Design review of the part built by this model. Coordinates are the model's own, in mm. Give positions to 0.01 mm unless a question says otherwise; leave off trailing zeros. Write each loop counter-clockwise with the first axis right and the second up, starting at its lowest first coordinate (ties: lowest second). Pieces come first, ordered by that corner, then holes. Notation, with made-up numbers: (14.25, -3.5) -> (67.25, -3.5) arc R18 ccw to (67.25, 31.5) -> close; hole circle Ø2 at (5, 9). An arc over 180 degrees is marked (long way). Return JSON: item names as keys, results as strings. Group by question number.
Autodesk Inventor part; units mm, degrees
ref_plane "YZ Plane" through (0, 0, 0) normal (1, 0, 0) x (0, 1, 0)
ref_plane "XZ Plane" through (0, 0, 0) normal (0, 1, 0) x (-1, 0, 0)
ref_plane "XY Plane" through (0, 0, 0) normal (0, 0, 1) x (1, 0, 0)
sketch "Sketch1" plane through (0, 0, 0) normal (0, 0, 1) x (1, 0, 0)
  line L0 (12.7, -4.7625) -> (-12.7, -4.7625)
  line L1 (-12.7, -4.7625) -> (-12.7, 4.7625)
  line L2 (-12.7, 4.7625) -> (12.7, 4.7625)
  line L3 (12.7, 4.7625) -> (12.7, -4.7625)
  line L4 (12.7, -4.7625) -> (-12.7, 4.7625) construction
  line L5 (-12.7, -4.7625) -> (12.7, 4.7625) construction
  line L6 (-12.7, 0) -> (12.7, 0) construction
  circle A0 centre (-7.1437, 0) radius 2.4892
  line L7 (0, -4.7625) -> (0, 4.7625) construction
  circle A1 centre (7.1437, 0) radius 2.4892
  point P0 (0, 0)
  point P1 (0, 0)
  dimension "d0" = 25.4
  dimension "d1" = 9.525
  dimension "d2" = 4.9784
  dimension "d3" = 7.1437
extrude "Extrusion1" add sketch "Sketch1" along normal blind 6.35
properties part number "Arms" material "Aluminum 6061"
Q1. Take a section at D-D, the plane y = 1.5. Give the boundary of the cut face in (x, z).
Q2. Take a section at B-B, the plane z = 3.5. Give the boundary of the cut face in (x, y).
Q3. Take a section at A-A, the plane y = 0. Give the boundary of the cut face in (x, z), plus the area to 3 significant figures.
Q4. Take a section at C-C, the plane x = 9. Give the boundary of the cut face in (y, z), plus the area to 3 significant figures.
Q5. For L1, parallel to Y at x = -7.25, z = 0.5; L2, parallel to X at y = -1.75, z = 1; L3, parallel to X at y = -2, z = 0.75, list the stretches that pass through material, from the lowest coordinate up. Write a range as from..to.
Q6. Insertion check: pin 1 (4 mm diameter, centred on x = 7.14, y = 0, fed in from -Z). The pin has a flat end and moves straight along its axis. Give the tip position at first contact, or say it passes through.
Q7. Mouldability with a two-part tool opening along Y and no side actions: class faces 1 (the face through (0, -4.762, 3)), 2 (the face through (0, 0, 6.35)), 3 (the face through (9.443, 0.953, 3.131)), 4 (the face through (0, 4.762, 3)) as +Y half, -Y half, draft (parallel to the pull), parting line (faces both ways), or undercut.
Final values:
{
 "1": {"outline": "(-12.7, 0) -> (-9.13, 0) -> (-9.13, 6.35) -> (-12.7, 6.35) -> close; (-5.16, 0) -> (5.16, 0) -> (5.16, 6.35) -> (-5.16, 6.35) -> close; (9.13, 0) -> (12.7, 0) -> (12.7, 6.35) -> (9.13, 6.35) -> close"},
 "2": {"outline": "(-12.7, -4.76) -> (12.7, -4.76) -> (12.7, 4.76) -> (-12.7, 4.76) -> close; hole circle Ø4.98 at (-7.14, 0); hole circle Ø4.98 at (7.14, 0)"},
 "3": {"outline": "(-12.7, 0) -> (-9.63, 0) -> (-9.63, 6.35) -> (-12.7, 6.35) -> close; (-4.65, 0) -> (4.65, 0) -> (4.65, 6.35) -> (-4.65, 6.35) -> close; (9.63, 0) -> (12.7, 0) -> (12.7, 6.35) -> (9.63, 6.35) -> close", "area": "98.1 mm²"},
 "4": {"outline": "(-4.76, 0) -> (-1.66, 0) -> (-1.66, 6.35) -> (-4.76, 6.35) -> close; (1.66, 0) -> (4.76, 0) -> (4.76, 6.35) -> (1.66, 6.35) -> close", "area": "39.4 mm²"},
 "5": {"L1": "y = -4.76..-2.49, 2.49..4.76", "L2": "x = -12.7..-8.91, -5.37..5.37, 8.91..12.7", "L3": "x = -12.7..-8.63, -5.66..5.66, 8.63..12.7"},
 "6": {"pin 1": "passes through"},
 "7": {"face 1": "-Y half", "face 2": "draft", "face 3": "undercut", "face 4": "+Y half"}
}
